Answer from the drawing. Dimensions are ordinates in mm from the lowest x, y and z of the part. A direction names the side the tool comes from. Give positions to 0.01 mm unless a question says otherwise; leave off trailing zeros. Order: outer loops, then holes, each group sorted by start corner. A loop starts at its lowest first (then second) coordinate and runs counter-clockwise, first axis right, second up. Notation, with made-up numbers: (80, 68.5) - (99, 68.5) arc R22 ccw to (99, 80.5) - close; hole circle Ø9 at (-4, 58). An arc over 180 degrees is marked (long way). One line per item, written item: value. Start each with the question number.
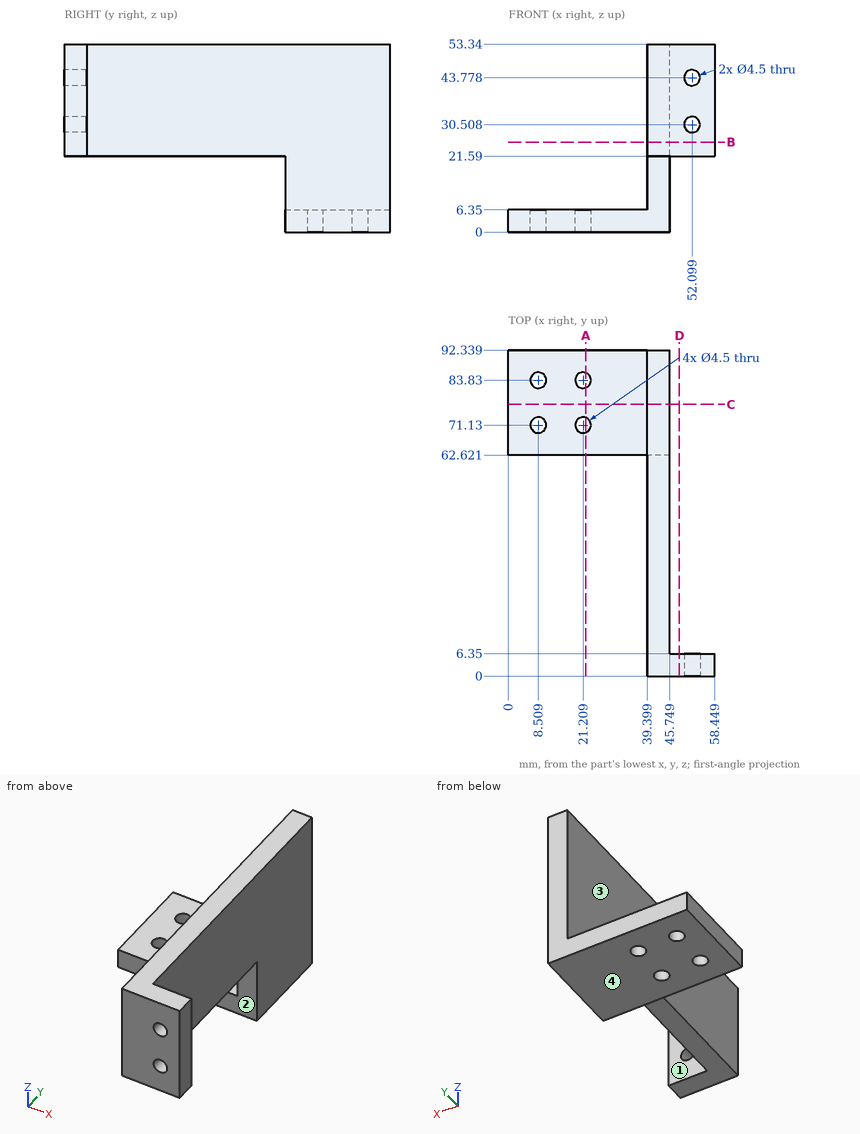
1) For the marked faces 1, 2, 3 and 4, determine the directions among +Z, -Z, +X, -X, +Y, -Y from which every point of the face is accessible in a straight line to the end or side of a thin tool.
2) Find the intervals of material crossed by probe 1 along X at (y, z) = (45.5, 27.5); probe 2 along Y at (x, z) = (40, 15.5); probe 3 along X at (y, z) = (4, 39), in increasing order. Write a range as from..to.
3) Section A-A on x = 22 is taken. Write down the section's boundary in (y, z).
4) Section D-D on x = 48.5 is taken. Write down the section's boundary in (y, z).
5) Section C-C on y = 77 is taken. Write down the section's boundary in (x, z).
6) Each of these flat-tipped pins is pushed along its axis until it touches: pin 1 (6 mm diameter, centred on x = 21.21, y = 83.83, fed in from +Z); pin 2 (5.5 mm diameter, centred on x = 47, y = 25.5, fed in from -Z); pin 3 (12 mm diameter, centred on x = 35, z = 27.5, fed in from -Y); pin 4 (5 mm diameter, centred on x = 52.1, z = 30.51, fed in from +Y). Where does it stop, or does it pass through?
7) Section B-B on z = 25.5 is taken. Write down the section's boundary in (x, y).
Solved:
1. face 1: +Z, -Z, +X, +Y
1. face 2: -Z, +X, -X, -Y
1. face 3: +Z, -X, +Y, -Y
1. face 4: -Z, +X, -X, +Y, -Y
2. probe 1: x = 39.4..45.75
2. probe 2: y = 62.62..92.34
2. probe 3: x = 39.4..58.45
3. outline: (62.62, 0) - (69.02, 0) - (69.02, 6.35) - (62.62, 6.35) - close; (73.24, 0) - (81.72, 0) - (81.72, 6.35) - (73.24, 6.35) - close; (85.94, 0) - (92.34, 0) - (92.34, 6.35) - (85.94, 6.35) - close
4. outline: (0, 21.59) - (6.35, 21.59) - (6.35, 53.34) - (0, 53.34) - close
5. outline: (0, 0) - (45.75, 0) - (45.75, 53.34) - (39.4, 53.34) - (39.4, 6.35) - (0, 6.35) - close
6. pin 1: stops at z = 6.35
6. pin 2: stops at z = 21.59
6. pin 3: stops at y = 0
6. pin 4: stops at y = 6.35
7. outline: (39.4, 0) - (58.45, 0) - (58.45, 6.35) - (45.75, 6.35) - (45.75, 92.34) - (39.4, 92.34) - close
